The figure shows three views and two pictorial views of one solid part (mm, origin at its lowest corner). Answer the questions. A direction names the side the tool comes from. Round coordinates to 2 decimals unless told otherwise and drop trailing zeros. Write each loop counter-clockwise with the first axis right and the second up, starting at its lowest first coordinate (ties: lowest second). Pieces come first, ordered by that corner, then holes. Notation, with made-up numbers: M 9.5,23 L 24.5,23 A19 ccw 24.5,45 Z; hole C 7.25,0.5 d8. An arc over 180 degrees is marked long. Answer in a Markdown table with one row per item.
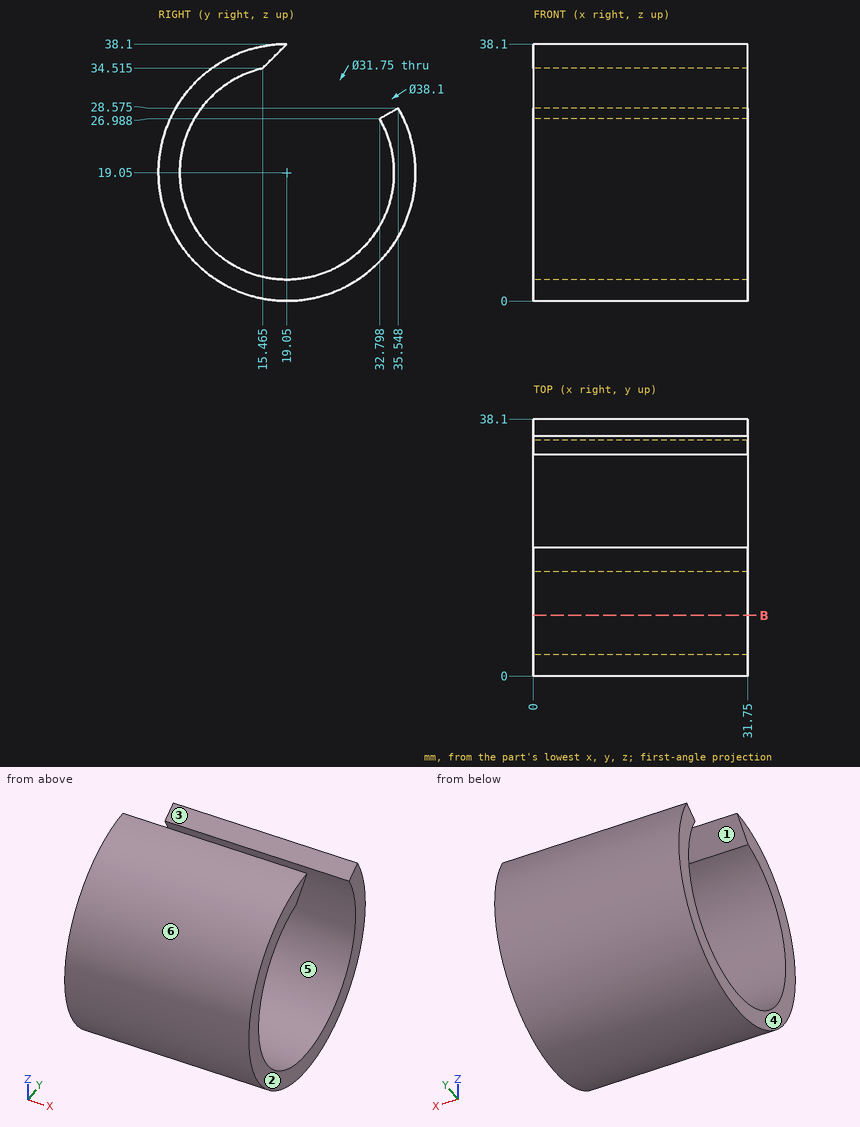
1. The part is cut by section B-B (y = 9). Determine the outline of the cut face in (x, z), plus the area to 3 significant figures.
Calculated:
| item | result |
|---|---|
| outline | M 0,2.87 L 31.75,2.87 L 31.75,6.76 L 0,6.76 Z; M 0,31.34 L 31.75,31.34 L 31.75,35.23 L 0,35.23 Z |
| area | 247 mm² |
2. Given pin 1 (1.5 mm diameter, centred on x = 12.5, z = 18.5, fed in from +Y); pin 2 (2 mm diameter, centred on x = 7, z = 30.5, fed in from +Y); pin 3 (3 mm diameter, centred on x = 10, y = 28.5, fed in from +Z) (1 decimal), each flat-ended and moving along its own axis, determine where each tip first touches the part or whether it passes through.
Calculated:
| item | result |
|---|---|
| pin 1 | stops at y = 38.1 |
| pin 2 | stops at y = 9.2 |
| pin 3 | stops at z = 7.6 |
3. Determine the mould class of the marked faces 4, 5 and 6 for opening direction Z: released by +Z, released by -Z, zero draft, split by the parting line, or undercut.
Calculated:
| item | result |
|---|---|
| face 4 | zero draft |
| face 5 | undercut |
| face 6 | split by the parting line |
4. Consider line 1 along Y through (x, z) = (12, 19.05) (1 decimal); line 2 along Z through (x, y) = (5, 12.5); line 3 along Y through (x, z) = (4.5, 5) (1 decimal). Determine where each line is inside the solid, lowest interval first. Write a range as from..to.
Calculated:
| item | result |
|---|---|
| line 1 | y = 0..3.2, 34.9..38.1 |
| line 2 | z = 1.16..4.59, 33.51..36.94 |
| line 3 | y = 6.2..11.7, 26.4..31.9 |
5. A tool of negligible diameter and unlimited length cuts with its end or side. For the marked faces 1, 2 and 3, from which of +Z, -Z, +X, -X, +Y, -Y can it reach the whole face along a straight path? Write none if from no direction.
Calculated:
| item | result |
|---|---|
| face 1 | +X, -X, +Y |
| face 2 | +Z, -Z, +X, +Y, -Y |
| face 3 | +Z, +X, -X |
